Work out the finished part from the listing and answer in its coordinate system (mm). A direction names the side the tool comes from. Round coordinates to 2 decimals unless told otherwise and drop trailing zeros. Write each loop counter-clockwise with the first axis right and the second up, starting at its lowest first coordinate (ties: lowest second). Pieces come first, ordered by that corner, then holes. Notation, with made-up numbers: (28.25, 35.25) - (68.25, 35.25) arc R22 ccw to (68.25, 71.25) - close; hole circle Ø3 at (29, 2.5). An arc over 180 degrees is marked (long way). Answer as a JSON object with one key per item and string values.
```python
from build123d import *

# Parameters (mm, degrees)
SKETCH1_R           = 4.4
BOSS_EXTRUDE1_DEPTH = 5
SKETCH2_W           = 92
SKETCH2_H           = 5
BOSS_EXTRUDE2_DEPTH = 20
FILLET1_R           = 10
SKETCH3_R           = 5
CUT_EXTRUDE1_DEPTH  = 5
CUT_EXTRUDE1_TAPER  = 24


with BuildPart() as part:
    # Sketch1 → Boss-Extrude1 (new body)
    with BuildSketch(Plane(origin=(0, 0, 0), x_dir=(1, 0, 0), z_dir=(0, 1, 0))):
        with BuildLine():
            Line((-36, 40), (36, 40))
            ThreePointArc((36, 40), (43.071067812, 37.071067812), (46, 30))
            Line((46, 30), (46, -30))
            ThreePointArc((46, -30), (43.071067812, -37.071067812), (36, -40))
            Line((36, -40), (-36, -40))
            ThreePointArc((-36, -40), (-43.071067812, -37.071067812), (-46, -30))
            Line((-46, -30), (-46, 30))
            ThreePointArc((-46, 30), (-43.071067812, 37.071067812), (-36, 40))
        make_face()
        with Locations((-26, -15)):
            Circle(SKETCH1_R, mode=Mode.SUBTRACT)
        with Locations((26, -15)):
            Circle(SKETCH1_R, mode=Mode.SUBTRACT)
    extrude(amount=-BOSS_EXTRUDE1_DEPTH)

    # Sketch2 → Boss-Extrude2 (add)
    with BuildSketch(Plane(origin=(0, 0, 0), x_dir=(1, 0, 0), z_dir=(0, 1, 0))):
        with Locations((0, 7.5)):
            Rectangle(SKETCH2_W, SKETCH2_H)
    extrude(amount=BOSS_EXTRUDE2_DEPTH)

    # Fillet1
    fillet1_edges = [part.edges().sort_by_distance(p)[0] for p in [
        (0, 0, -5),
    ]]
    fillet(fillet1_edges, radius=FILLET1_R)

    # Sketch3 → Cut-Extrude1 (cut)
    with BuildSketch(Plane.XZ.offset(5)):
        with Locations((-26, -24)):
            Circle(SKETCH3_R)
        with Locations((26, -24)):
            Circle(SKETCH3_R)
    extrude(amount=-CUT_EXTRUDE1_DEPTH, taper=CUT_EXTRUDE1_TAPER, mode=Mode.SUBTRACT)


solid = part.part
```
Item 1: A cutting plane is placed at D-D (y = 14.75). Write down the section's boundary in (x, z).
Results found:
{"outline": "(-46, -10) - (46, -10) - (46, -5) - (-46, -5) - close"}
Item 2: Consider line 1 along X through (y, z) = (-2.8, 15); line 2 along Z through (x, y) = (26, -2.55); line 3 along Z through (x, y) = (29, 17.5). Determine where each line is inside the solid, lowest interval first.
Results found:
{"line 1": "-46 to -30.4, -21.6 to 21.6, 30.4 to 46", "line 2": "-40 to -27.91, -20.09 to 10.6, 19.4 to 40", "line 3": "-10 to -5"}
Item 3: Determine the mould class of faces 1 (the flat face through (-46, 1, -2)), 2 (the cylindrical face through (42.99, -2.46, -37.15)), 3 (the conical face through (-23, -0.8, -23.1)), 4 (the cylindrical face through (-23.635, -2.465, 11.29)) for opening direction Z: pulls with the +Z half, pulls with the -Z half, needs draft (parallel to the pull), parting line crosses it, or undercut.
Results found:
{"face 1": "needs draft", "face 2": "pulls with the -Z half", "face 3": "undercut", "face 4": "undercut"}
Item 4: A cutting plane is placed at B-B (y = -1.5). Write down the section's boundary in (x, z).
Results found:
{"outline": "(-46, -30) arc R10 ccw to (-36, -40) - (36, -40) arc R10 ccw to (46, -30) - (46, 30) arc R10 ccw to (36, 40) - (-36, 40) arc R10 ccw to (-46, 30) - close; hole circle Ø8.8 at (-26, 15); hole circle Ø6.88 at (-26, -24); hole circle Ø8.8 at (26, 15); hole circle Ø6.88 at (26, -24)"}
Item 5: A cutting plane is placed at A-A (z = 15). Write down the section's boundary in (x, y).
Results found:
{"outline": "(-46, -5) - (-30.4, -5) - (-30.4, 0) - (-46, 0) - close; (-21.6, -5) - (21.6, -5) - (21.6, 0) - (-21.6, 0) - close; (30.4, -5) - (46, -5) - (46, 0) - (30.4, 0) - close"}
Item 6: For faces 5 (the cylindrical face through (43.15, -2.46, 36.99)), 6 (the flat face through (1, 0, -25)), 7 (the flat face through (1, 0, 22)), determine the directions among +Z, -Z, +X, -X, +Y, -Y from which every point of the face is accessible in a straight line to the end or side of a thin tool.
Results found:
{"face 5": "+Z, +X, +Y, -Y", "face 6": "-Z, +X, -X, +Y", "face 7": "+Z, +X, -X, +Y"}
Item 7: Each of these flat-tipped pins is pushed along its axis until it touches: P1, Ø10.5, axis at x = -4, z = 28, coming from the +Y side; P2, Ø12, axis at y = 10, z = -14.5, coming from the -X side; P3, Ø11, axis at x = -12.5, y = 17, coming from the +Z side; P4, Ø10, axis at x = -29, y = 16, coming from the -Z side. Where does it stop, or does it pass through?
Results found:
{"P1": "y = 0", "P2": "x = -46", "P3": "z = -5", "P4": "z = -10"}
Item 8: A cutting plane is placed at C-C (x = 20). Write down the section's boundary in (y, z).
Results found:
{"outline": "(-5, -40) - (0, -40) - (0, -10) - (20, -10) - (20, -5) - (10, -5) arc R10 cw to (0, 5) - (0, 40) - (-5, 40) - close"}
